```python
from build123d import *

# Parameters (mm, degrees)
F0_W            = 20
F0_H            = 40
F1_DEPTH        = 40
F2_R            = 5
F3_R            = 6
F4_R            = 2
F5_R            = 5.975
F6_DEPTH        = 40.001
F8_D            = 4
F8_DEPTH        = 40
F8_TIP          = 1.2017212381
F10_D           = 4
F10_DEPTH       = 12
F10_TIP         = 1.2017212381
F12_D           = 4
F12_DEPTH       = 12
F12_TIP         = 1.2017212381
F14_D           = 4
F14_DEPTH       = 12
F14_CSINK_D     = 10
F14_CSINK_ANGLE = 90
F14_TIP         = 1.2017212381


with BuildPart() as f1:
    # F0 (on Top) → F1 (new body)
    with BuildSketch(Plane.XY):
        Polygon((-17.5, 30.3108891325), (17.5, 30.3108891325), (31.75, 54.9926131403), (14.4294919243, 64.9926131403), (51.4294919243, 129.0784930204), (46.2333395016, 132.0784930204), (36.8527810232, 115.8308891325), (-36.8527810232, 115.8308891325), (-46.2333395016, 132.0784930204), (-51.4294919243, 129.0784930204), (-14.4294919243, 64.9926131403), (-31.75, 54.9926131403), align=None)
        with Locations((0, 56.1808891325)):
            Rectangle(F0_W, F0_H, mode=Mode.SUBTRACT)
        Polygon((34.5433799465, 111.8308891325), (18.5796450034, 84.1808891325), (-18.5796450034, 84.1808891325), (-34.5433799465, 111.8308891325), align=None, mode=Mode.SUBTRACT)
    extrude(amount=F1_DEPTH)

    # F2
    f2_edges = [f1.edges().sort_by_distance(p)[0] for p in [
        (-17.5, 30.310889, 20),
        (17.5, 30.310889, 20),
    ]]
    fillet(f2_edges, radius=F2_R)

    # F3
    f3_edges = [f1.edges().sort_by_distance(p)[0] for p in [
        (18.579645, 84.180889, 20),
        (-18.579645, 84.180889, 20),
        (-36.852781, 115.830889, 20),
        (36.852781, 115.830889, 20),
    ]]
    fillet(f3_edges, radius=F3_R)

    # F4
    f4_edges = [f1.edges().sort_by_distance(p)[0] for p in [
        (34.54338, 111.830889, 20),
        (-34.54338, 111.830889, 20),
    ]]
    fillet(f4_edges, radius=F4_R)

    # F5 (on face) → F6 (cut, through all)
    with BuildSketch(Plane.XY.offset(40)):
        with Locations((-18.8069092991, 51.5245224395)):
            Circle(F5_R)
        with Locations((18.8069092991, 51.5245224395)):
            Circle(F5_R)
    extrude(amount=-F6_DEPTH, mode=Mode.SUBTRACT)

    # F8
    with Locations(Plane(origin=(0, 115.8308891325, 0), x_dir=(-1, 0, 0), z_dir=(0, 1, 0))):
        with Locations((0, 20)):
            Hole(F8_D / 2, depth=F8_DEPTH)
            with Locations((0, 0, -(F8_DEPTH + F8_TIP / 2))):  # 118° drill point
                Cone(0, F8_D / 2, F8_TIP, mode=Mode.SUBTRACT)

    # F10
    with Locations(Plane(origin=(-17.3205080757, 10, 0), x_dir=(0.5, 0.8660254038, 0), z_dir=(0.8660254038, -0.5, 0))):
        with Locations((129.5, 32), (92.5, 32), (92.5, 8), (129.5, 8)):
            Hole(F10_D / 2, depth=F10_DEPTH)
            with Locations((0, 0, -(F10_DEPTH + F10_TIP / 2))):  # 118° drill point
                Cone(0, F10_D / 2, F10_TIP, mode=Mode.SUBTRACT)

    # F12
    with Locations(Plane(origin=(17.3205080757, 10, 0), x_dir=(0.5, -0.8660254038, 0), z_dir=(-0.8660254038, -0.5, 0))):
        with Locations((-129.5, 32), (-129.5, 8), (-92.5, 8), (-92.5, 32)):
            Hole(F12_D / 2, depth=F12_DEPTH)
            with Locations((0, 0, -(F12_DEPTH + F12_TIP / 2))):  # 118° drill point
                Cone(0, F12_D / 2, F12_TIP, mode=Mode.SUBTRACT)

    # F14
    with Locations(Plane.XZ.offset(-30.3108891325)):
        with Locations((0, 30), (0, 10)):
            CounterSinkHole(F14_D / 2, F14_CSINK_D / 2, depth=F14_DEPTH, counter_sink_angle=F14_CSINK_ANGLE)
            with Locations((0, 0, -(F14_DEPTH + F14_TIP / 2))):  # 118° drill point
                Cone(0, F14_D / 2, F14_TIP, mode=Mode.SUBTRACT)


solid = f1.part
```
Can you work these out from the model? Positions are in its coordinate system, mm. A direction names the side the tool comes from. Give positions to 0.01 mm unless a question says otherwise; leave off trailing zeros. Order: outer loops, then holes, each group sorted by start corner. A loop starts at its lowest first (then second) coordinate and runs counter-clockwise, first axis right, second up. Notation, with made-up numbers: M 72,-36.5 L 99,-36.5 A31 ccw 99,2.5 Z; hole C -24.75,80 d4. An arc over 180 degrees is marked long. Write item = value, one per line. Start each with the question number.
Q1. Suppose I cut it at B-B (y = 117.5). Write out the boundary of the cut face in (x, z).
Q2. Will these pins go through, and if not, where does the flat tip stop? pin 1 Ø22 at (x, z) = (-4.5, 20.5) entering from +Y; pin 2 Ø10 at (x, z) = (-0.5, 28) entering from -Y; pin 3 Ø9.5 at (x, y) = (-18.81, 51.52) entering from -Z; pin 4 Ø12 at (y, z) = (104, 31.5) entering from -X.
Q3. Suppose I cut it at A-A (x = 0). Count the separate pieces of the cut face and the enclosed holes in it, plus the area to 3 significant figures.
Q4. Suppose I cut it at C-C (y = 77.5). Write out the boundary of the cut face in (x, z).
Q5. I need wall thicknesses on probe 1 along Y at (x, z) = (-4.5, 22); probe 2 along Z at (x, y) = (0, 79); probe 3 along Y at (x, z) = (14.5, 34). Which ranges of each line are inside material? Lowest first, please. Write a range as [from, to].
Q6. We'd pull the mould along Z, two halves only. Please class faces 4 (the flat face through (0, 81, 40)), 5 (the cylindrical face through (18.077, 84.963, 20.28)), 6 (the cylindrical face through (-26.078, 91.253, 30.048)): pulls with the +Z half, pulls with the -Z half, needs draft (parallel to the pull), parting line crosses it, or undercut.
Q7. For faces 1 (the flat face through (23.211, 59.923, 19.72)), 2 (the flat face through (26.65, 98.16, 19.72)), 3 (the cylindrical face through (0, 80, 22)), which set-ups out of +Z, -Z, +X, -X, +Y, -Y let a thin tool reach every point of the face, with its end or its side?
Check result:
q1.outline = M -44.74,0 L -37.54,0 L -37.54,40 L -44.74,40 Z; M 37.54,0 L 44.74,0 L 44.74,40 L 37.54,40 Z
q2.pin_1 = 115.83
q2.pin_2 = 30.31
q2.pin_3 = through
q2.pin_4 = -40.41
q3.separate_pieces = 7
q3.enclosed_holes = 0
q3.area = 602 mm2
q4.outline = M -21.65,0 L 21.65,0 L 21.65,40 L -21.65,40 Z; hole C 0,20 d4
q5.probe_1 = [30.31, 36.18], [76.18, 84.18], [111.83, 115.83]
q5.probe_2 = [0, 18], [22, 40]
q5.probe_3 = [30.31, 47.38], [55.67, 64.95], [65.11, 84.18], [111.83, 115.83]
q6.face_4 = pulls with the +Z half
q6.face_5 = needs draft
q6.face_6 = undercut
q7.face_1 = +Z, -Z, +X
q7.face_2 = +Z, -Z
q7.face_3 = +Y
